Answer from the drawing. Dimensions are ordinates in mm from the lowest x, y and z of the part. A direction names the side the tool comes from. Coordinates: 2 decimals unless noted, no trailing zeros. Loops run counter-clockwise (first coordinate to the right, second up) from the corner with the lowest first, then second, coordinate; pieces in that order, holes last. Notation, with made-up numbers: (-24, 70.25) - (2, 70.25) arc R11 cw to (2, 88.25) - close; hole circle Ø8 at (41, 18). An arc over 180 degrees is marked (long way). Use one line per item in the form item = value. Start each with the question number.
1) A cutting plane is placed at A-A (y = 5.5). Give the vertices of the cut face in (x, z), and give its area (3 significant figures).
2) Consider line 1 (Z direction, x = 11, y = 1.25); line 2 (X direction, y = 3.75, z = 14). Determine where each line is inside the solid, lowest interval first.
3) The mould has two halves that part along X. Classify the marked faces 3, 4 and 5: released by +X, released by -X, zero draft, split by the parting line, or undercut.
4) A cutting plane is placed at C-C (x = 2.75). Give the vertices of the cut face in (y, z).
5) This flat-tipped pin is pushed along its axis until it touches: P1, Ø7, axis at x = 7, z = 8.5, coming from the +Y side. Where does it stop, or does it pass through?
6) Which of the six approach directions +Z, -Z, +X, -X, +Y, -Y give full straight-line access (tool end or side, diameter ignored) to the marked faces 1 and 2?
7) A cutting plane is placed at B-B (z = 2.25). Give the vertices of the cut face in (x, y).
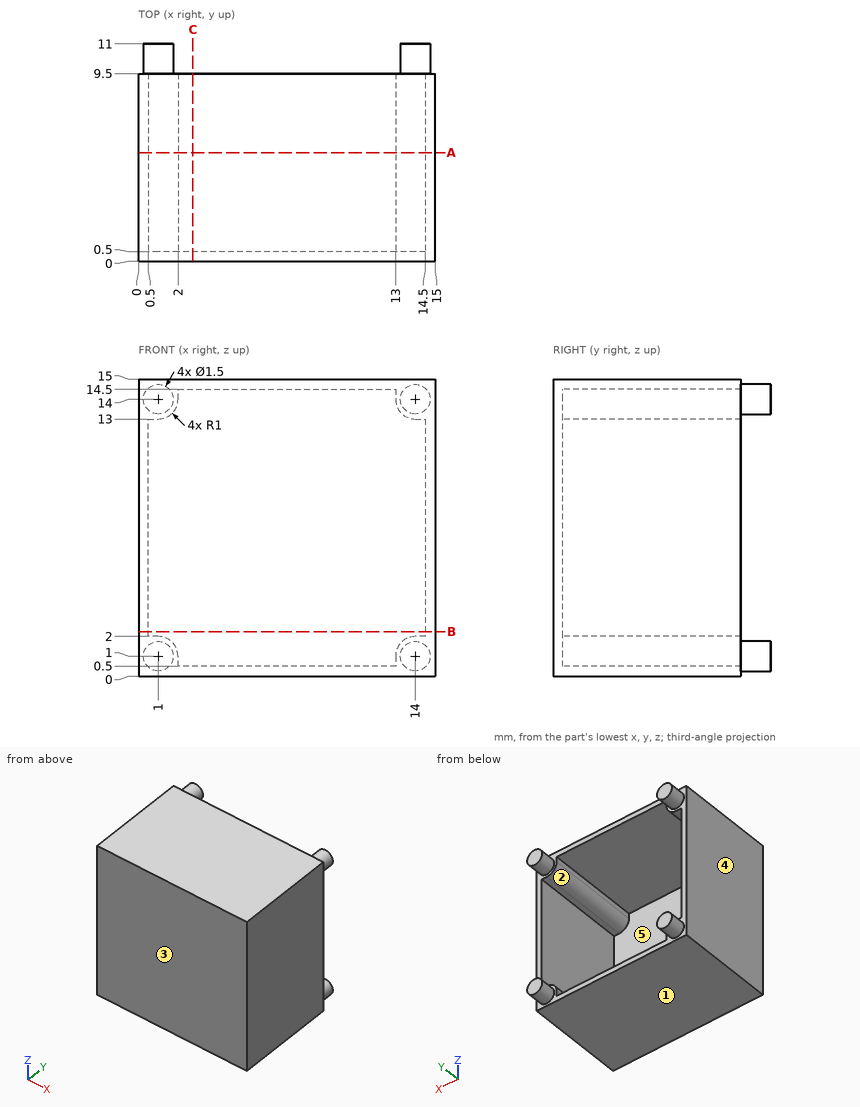
Found:
q1.outline = (0, 0) - (15, 0) - (15, 15) - (0, 15) - close; hole (0.5, 2) - (1, 2) arc R1 cw to (2, 1) - (2, 0.5) - (13, 0.5) - (13, 1) arc R1 cw to (14, 2) - (14.5, 2) - (14.5, 13) - (14, 13) arc R1 cw to (13, 14) - (13, 14.5) - (2, 14.5) - (2, 14) arc R1 cw to (1, 13) - (0.5, 13) - close
q1.area = 37.1 mm^2
q2.line_1 = 0 to 0.5, 14.5 to 15
q2.line_2 = 0 to 2, 13 to 15
q3.face_3 = zero draft
q3.face_4 = released by -X
q3.face_5 = undercut
q4.outline = (0, 0) - (9.5, 0) - (9.5, 0.5) - (0.5, 0.5) - (0.5, 14.5) - (9.5, 14.5) - (9.5, 15) - (0, 15) - close
q5.P1 = 0.5
q6.face_1 = -Z, +X, -X, +Y, -Y
q6.face_2 = +Y
q7.outline = (0, 0) - (15, 0) - (15, 9.5) - (14.5, 9.5) - (14.5, 0.5) - (0.5, 0.5) - (0.5, 9.5) - (0, 9.5) - close
